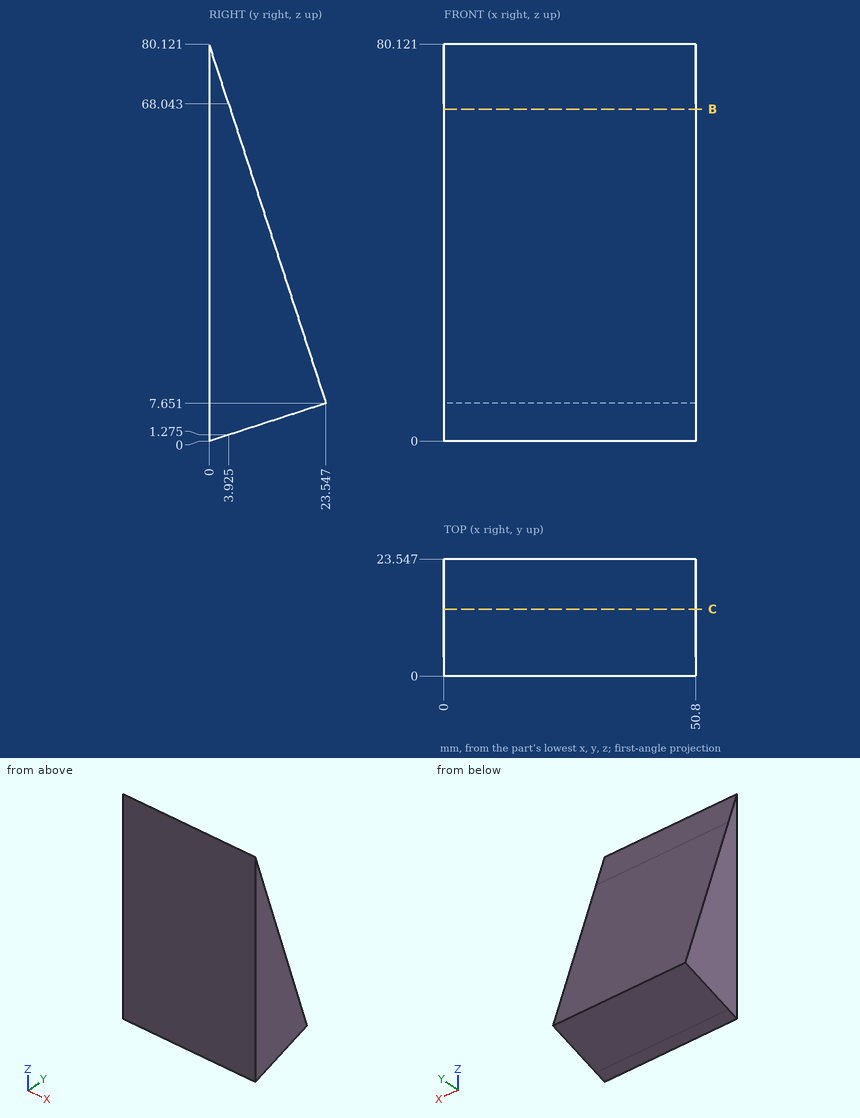
Verification items for this drawing (mm, ordinates from the low corner). Coordinates: 2 decimals unless noted, no trailing zeros. Write each loop counter-clockwise with the first axis right and the second up, starting at its lowest first coordinate (ties: lowest second). Pieces come first, ordered by that corner, then holes. Notation, with made-up numbers: (59, -26) -> (111, -26) arc R13 ccw to (111, -4) -> close; hole circle Ø5 at (-11.75, 53.5). An arc over 180 degrees is marked (long way). One line per item, written item: value. Start each with the question number.
Q1. Cross-section at C-C on y = 13.5. Enter the section's corners in (x, z).
Q2. Cross-section at B-B on z = 67. Enter the section's corners in (x, y).
Q3. Go/stop test with flat-tipped pins: P1, Ø1.5, axis at x = 29, z = 41.5, coming from the +Y side; P2, Ø3, axis at x = 36, y = 5.5, coming from the -Z side; P3, Ø5, axis at x = 41, z = 10.5, coming from the +Y side. Record where each tip stops, or that it passes through.
Q4. Thickness scan on L1, parallel to Y at x = 45, z = 16 (1 decimal); L2, parallel to Y at x = 36.5, z = 67.5. Record the ranges inside material, lowest first. Write a range as from..to.
Checked values:
1. outline: (0, 4.39) -> (50.8, 4.39) -> (50.8, 38.57) -> (0, 38.57) -> close
2. outline: (0, 0) -> (50.8, 0) -> (50.8, 4.26) -> (0, 4.26) -> close
3. P1: stops at y = 12.79
3. P2: stops at z = 1.3
3. P3: stops at y = 23.43
4. L1: y = 0..20.8
4. L2: y = 0..4.1
